Input: part model. Units: mm. Frame: model coordinates. A direction names the side the tool comes from. Give positions to 0.01 mm unless a question says otherwise; leave off trailing zeros. Loops run counter-clockwise (first coordinate to the right, second up) from the corner with the lowest first, then second, coordinate; pieces in that order, holes last. Notation, with made-up numbers: M 5.25,84 L 51.25,84 A11 cw 51.25,104 Z; hole C -17.75,61 d5. An arc over 180 degrees is marked long. Use CSV: the item, a comma, the result in double quotes. Start each with the question number.
from build123d import *

# Parameters (mm, degrees)
F0_R     = 12.5
F1_DEPTH = 25
F0_R_2   = 25
F2_DEPTH = 50
F0_R_3   = 37.5
F3_DEPTH = 75
F0_R_4   = 50
F4_DEPTH = 100
F5_D     = 5


with BuildPart() as f1:
    # F0 (on Top) → F1 (new body)
    with BuildSketch(Plane.XY):
        Circle(F0_R)
    extrude(amount=F1_DEPTH)

    # F0 (on Top) → F2 (join)
    with BuildSketch(Plane.XY):
        Circle(F0_R_2)
        Circle(F0_R, mode=Mode.SUBTRACT)
    extrude(amount=F2_DEPTH)

    # F0 (on Top) → F3 (join)
    with BuildSketch(Plane.XY):
        Circle(F0_R_3)
        Circle(F0_R_2, mode=Mode.SUBTRACT)
    extrude(amount=F3_DEPTH)

    # F0 (on Top) → F4 (join)
    with BuildSketch(Plane.XY):
        Circle(F0_R_4)
        Circle(F0_R_3, mode=Mode.SUBTRACT)
    extrude(amount=F4_DEPTH)

    # F5 (through all)
    with Locations(Plane(origin=(0, 0, 0), x_dir=(1, 0, 0), z_dir=(0, 0, -1))):
        with Locations((0, 0)):
            Hole(F5_D / 2)


solid = f1.part
Item 1: Section D-D (x = 16.5). Output: boundary loops of the cut face in (y, z), then the cut area to 3 significant figures.
Item 2: Section C-C (z = 67). Output: boundary loops of the cut face in (x, y).
Item 3: Section A-A (y = 0). Output: boundary loops of the cut face in (x, z), then the cut area to 4 significant figures.
Item 4: Set-up query: faces 4 (the flat face through (-1, -10, 0)), 5 (the cylindrical face through (11.923, 3.755, 37.325)). Return all of +Z, -Z, +X, -X, +Y, -Y with unobstructed straight access to the full face (end or side cutting, diameter ignored); none if empty.
Item 5: First-contact query: pin 1 Ø2 at (y, z) = (28.5, 34.5) entering from -X; pin 2 Ø4 at (x, z) = (-31.5, 52.5) entering from -Y; pin 3 Ø12.5 at (x, y) = (5, 1.5) entering from +Z. Flat tips, straight axial feed; report the tip coordinate or a pass-through.
Item 6: Mould query, pull axis X, two halves, no side actions, for faces 1 (the flat face through (7, 37, 100)), 2 (the cylindrical face through (47.69, 15.02, 49.3)), 3 (the cylindrical face through (23.846, 7.509, 62.325)). Classes: +X half, -X half, draft (parallel to the pull), parting line (faces both ways), or undercut.
Item 7: Material intervals for line 1 (Y direction, x = 0, z = 33); line 2 (Y direction, x = 0, z = 85.75); line 3 (Z direction, x = 34.5, y = -13), sorted ascending.
Recorded:
1,outline,"M -47.2,0 L 47.2,0 L 47.2,100 L 33.67,100 L 33.67,75 L 18.78,75 L 18.78,50 L -18.78,50 L -18.78,75 L -33.67,75 L -33.67,100 L -47.2,100 Z"
1,area,"6,820 mm²"
2,outline,"C 0,0 d100; hole C 0,0 d50"
3,outline,"M -50,0 L -2.5,0 L -2.5,25 L -12.5,25 L -12.5,50 L -25,50 L -25,75 L -37.5,75 L -37.5,100 L -50,100 Z; M 2.5,0 L 50,0 L 50,100 L 37.5,100 L 37.5,75 L 25,75 L 25,50 L 12.5,50 L 12.5,25 L 2.5,25 Z"
3,area,"6,125 mm²"
4,face 4,"-Z, +X, -X, +Y, -Y"
4,face 5,"+Z"
5,pin 1,"x = -41.76"
5,pin 2,"y = -40.37"
5,pin 3,"z = 25"
6,face 1,"draft"
6,face 2,"parting line"
6,face 3,"undercut"
7,line 1,"-50 to -12.5, 12.5 to 50"
7,line 2,"-50 to -37.5, 37.5 to 50"
7,line 3,"0 to 75"
